from build123d import *

# Parameters (mm, degrees)
BOSS_EXTRUDE1_DEPTH = 80
SHELL1_T            = -3
SKETCH3_W           = 46
SKETCH3_H           = 47
BOSS_EXTRUDE2_DEPTH = 17
SKETCH4_W           = 10.2
SKETCH4_H           = 10.2
CUT_EXTRUDE1_DEPTH  = 20
SKETCH6_W           = 15
SKETCH6_H           = 12.8
CUT_EXTRUDE2_DEPTH  = 3
SKETCH7_W           = 40.4
SKETCH7_H           = 50
CUT_EXTRUDE3_DEPTH  = 5
FILLET1_R           = 4
CUT_EXTRUDE7_DEPTH  = 47
SKETCH13_R          = 1.5
CUT_EXTRUDE8_DEPTH  = 25
SKETCH14_R          = 3.1
CUT_EXTRUDE9_DEPTH  = 2
SKETCH17_W          = 45
SKETCH17_H          = 5
BOSS_EXTRUDE5_DEPTH = 74
CUT_EXTRUDE10_REACH = 126.093
SKETCH18_W          = 54
SKETCH18_H          = 45
CUT_EXTRUDE11_REACH = 126.093
SKETCH19_R          = 1.45
BOSS_EXTRUDE6_DEPTH = 47
SKETCH22_R          = 1.45
CUT_EXTRUDE12_DEPTH = 135.415364765
CUT_EXTRUDE13_REACH = 126.857
SKETCH24_R          = 3.7
SKETCH24_W          = 2
SKETCH24_H          = 3
BOSS_EXTRUDE7_DEPTH = 74
SKETCH27_R          = 1.5
CUT_EXTRUDE14_DEPTH = 10
CUT_EXTRUDE15_START = -3
CUT_EXTRUDE15_DEPTH = 32
CUT_EXTRUDE16_DEPTH = 30
BOSS_EXTRUDE8_DEPTH = 20
SKETCH31_R          = 1.5
CUT_EXTRUDE17_DEPTH = 123.649786567
CUT_EXTRUDE18_DEPTH = 15
CUT_EXTRUDE19_REACH = 126.093
SKETCH33_W          = 10
SKETCH33_H          = 5
SKETCH34_R          = 1.6
CUT_EXTRUDE20_DEPTH = 135.415364765
CUT_EXTRUDE22_DEPTH = 14


with BuildPart() as part:
    # Sketch2 → Boss-Extrude1 (new body)
    with BuildSketch(Plane(origin=(0, 0, 0), x_dir=(0, 0, -1), z_dir=(1, 0, 0))):
        Polygon((-27.320490368, 20.998248687), (-27.320490368, -29.001751313), (12.679509632, -29.001751313), (12.679509632, -48.511383538), (27.679509632, -48.511383538), (82.679509632, 0.998248687), (82.679509632, 20.998248687), align=None)
    extrude(amount=BOSS_EXTRUDE1_DEPTH)

    # Shell1
    shell1_openings = [part.faces().sort_by_distance(p)[0] for p in [
        (40, 20.998248687, -27.679509632),
    ]]
    offset(amount=SHELL1_T, openings=shell1_openings, kind=Kind.INTERSECTION)

    # Sketch3 → Boss-Extrude2 (add)
    with BuildSketch(Plane(origin=(0, 0, 24.320490368), x_dir=(-1, 0, 0), z_dir=(0, 0, -1))):
        with Locations((-40, -2.501751313)):
            Rectangle(SKETCH3_W, SKETCH3_H)
    extrude(amount=BOSS_EXTRUDE2_DEPTH)

    # Sketch4 → Cut-Extrude1 (cut)
    with BuildSketch(Plane.XY.offset(27.320490368)):
        with Locations((40, -4.001751313)):
            Rectangle(SKETCH4_W, SKETCH4_H)
    extrude(amount=-CUT_EXTRUDE1_DEPTH, mode=Mode.SUBTRACT)

    # Sketch6 → Cut-Extrude2 (cut)
    with BuildSketch(Plane.XZ.offset(29.001751313)):
        with Locations((40, 0.920490368)):
            Rectangle(SKETCH6_W, SKETCH6_H)
    extrude(amount=-CUT_EXTRUDE2_DEPTH, mode=Mode.SUBTRACT)

    # Sketch7 → Cut-Extrude3 (cut)
    with BuildSketch(Plane.XY.offset(27.320490368)):
        with Locations((40, -4.001751313)):
            Rectangle(SKETCH7_W, SKETCH7_H)
    extrude(amount=-CUT_EXTRUDE3_DEPTH, mode=Mode.SUBTRACT)

    # Fillet1
    fillet1_edges = [part.edges().sort_by_distance(p)[0] for p in [
        (80, -4.001751313, 27.320490368),
        (19.8, -4.001751313, 27.320490368),
        (0, -4.001751313, 27.320490368),
        (60.2, -4.001751313, 27.320490368),
    ]]
    fillet(fillet1_edges, radius=FILLET1_R)

    # Sketch12 → Cut-Extrude7 (cut)
    with BuildSketch(Plane(origin=(0, 20.998248687, 0), x_dir=(1, 0, 0), z_dir=(0, 1, 0))):
        Polygon((33, -7.320490368), (19.8, -12.320490368), (17, -24.320490368), (17, -7.320490368), align=None)
        Polygon((47, -7.320490368), (63, -7.320490368), (63, -24.320490368), (60.2, -12.320490368), align=None)
    extrude(amount=-CUT_EXTRUDE7_DEPTH, mode=Mode.SUBTRACT)

    # Sketch13 → Cut-Extrude8 (cut)
    with BuildSketch(Plane(origin=(0, 20.998248687, 0), x_dir=(1, 0, 0), z_dir=(0, 1, 0))):
        with Locations(Location((26, -17.320490368, 0), (0, 0, 270))):
            Circle(SKETCH13_R)
        with Locations(Location((54, -17.320490368, 0), (0, 0, 270))):
            Circle(SKETCH13_R)
    extrude(amount=-CUT_EXTRUDE8_DEPTH, mode=Mode.SUBTRACT)

    # Sketch14 → Cut-Extrude9 (cut)
    with BuildSketch(Plane(origin=(0, 20.998248687, 0), x_dir=(1, 0, 0), z_dir=(0, 1, 0))):
        with Locations(Location((26, -17.320490368, 0), (0, 0, 270))):
            Circle(SKETCH14_R)
        with Locations(Location((54, -17.320490368, 0), (0, 0, 270))):
            Circle(SKETCH14_R)
    extrude(amount=-CUT_EXTRUDE9_DEPTH, mode=Mode.SUBTRACT)

    # Sketch17 → Boss-Extrude5 (add)
    with BuildSketch(Plane.ZY.offset(-77)):
        with Locations((-23.179509632, -4.501751313)):
            Rectangle(SKETCH17_W, SKETCH17_H)
    extrude(amount=BOSS_EXTRUDE5_DEPTH)

    # Sketch18 → Cut-Extrude10 (cut, up to next)
    with BuildSketch(Plane(origin=(0, -2.001751313, 0), x_dir=(1, 0, 0), z_dir=(0, 1, 0)), mode=Mode.PRIVATE) as cut_extrude10_sk1:
        with Locations((40, 23.179509632)):
            Rectangle(SKETCH18_W, SKETCH18_H)
    cut_extrude10_tool1 = extrude(cut_extrude10_sk1.sketch, amount=-CUT_EXTRUDE10_REACH, mode=Mode.PRIVATE) & part.part
    add(cut_extrude10_tool1.solids().sort_by_distance((40, -2.001751, -23.17951))[0], mode=Mode.SUBTRACT)

    # Sketch19 → Cut-Extrude11 (cut, up to next)
    with BuildSketch(Plane(origin=(0, -2.001751313, 0), x_dir=(1, 0, 0), z_dir=(0, 1, 0)), mode=Mode.PRIVATE) as cut_extrude11_sk1:
        with Locations(Location((72, 37.179509632, 0), (0, 0, 270))):
            Circle(SKETCH19_R)
    cut_extrude11_tool1 = extrude(cut_extrude11_sk1.sketch, amount=-CUT_EXTRUDE11_REACH, mode=Mode.PRIVATE) & part.part
    # Sketch19 → Cut-Extrude11 (cut, up to next)
    with BuildSketch(Plane(origin=(0, -2.001751313, 0), x_dir=(1, 0, 0), z_dir=(0, 1, 0)), mode=Mode.PRIVATE) as cut_extrude11_sk2:
        with Locations(Location((72, 6.179509632, 0), (0, 0, 270))):
            Circle(SKETCH19_R)
    cut_extrude11_tool2 = extrude(cut_extrude11_sk2.sketch, amount=-CUT_EXTRUDE11_REACH, mode=Mode.PRIVATE) & part.part
    # Sketch19 → Cut-Extrude11 (cut, up to next)
    with BuildSketch(Plane(origin=(0, -2.001751313, 0), x_dir=(1, 0, 0), z_dir=(0, 1, 0)), mode=Mode.PRIVATE) as cut_extrude11_sk3:
        with Locations(Location((8, 33.179509632, 0), (0, 0, 270))):
            Circle(SKETCH19_R)
    cut_extrude11_tool3 = extrude(cut_extrude11_sk3.sketch, amount=-CUT_EXTRUDE11_REACH, mode=Mode.PRIVATE) & part.part
    # Sketch19 → Cut-Extrude11 (cut, up to next)
    with BuildSketch(Plane(origin=(0, -2.001751313, 0), x_dir=(1, 0, 0), z_dir=(0, 1, 0)), mode=Mode.PRIVATE) as cut_extrude11_sk4:
        with Locations(Location((8, 6.179509632, 0), (0, 0, 270))):
            Circle(SKETCH19_R)
    cut_extrude11_tool4 = extrude(cut_extrude11_sk4.sketch, amount=-CUT_EXTRUDE11_REACH, mode=Mode.PRIVATE) & part.part
    add(cut_extrude11_tool1.solids().sort_by_distance((72, -2.001751, -37.17951))[0], mode=Mode.SUBTRACT)
    add(cut_extrude11_tool2.solids().sort_by_distance((72, -2.001751, -6.17951))[0], mode=Mode.SUBTRACT)
    add(cut_extrude11_tool3.solids().sort_by_distance((8, -2.001751, -33.17951))[0], mode=Mode.SUBTRACT)
    add(cut_extrude11_tool4.solids().sort_by_distance((8, -2.001751, -6.17951))[0], mode=Mode.SUBTRACT)

    # Sketch21 → Boss-Extrude6 (add)
    with BuildSketch(Plane(origin=(0, -26.001751313, 0), x_dir=(1, 0, 0), z_dir=(0, 1, 0))):
        Polygon((3, -24.320490368), (3, -14.320490368), (19.333333333, -14.320490368), (17, -24.320490368), align=None)
    extrude(amount=BOSS_EXTRUDE6_DEPTH)

    # Sketch22 → Cut-Extrude12 (cut, through all)
    with BuildSketch(Plane(origin=(0, 20.998248687, 0), x_dir=(1, 0, 0), z_dir=(0, 1, 0))):
        with Locations(Location((10, -19.320490368, 0), (0, 0, 270))):
            Circle(SKETCH22_R)
    extrude(amount=-CUT_EXTRUDE12_DEPTH, mode=Mode.SUBTRACT)

    # Sketch24 → Cut-Extrude13 (cut, up to next)
    with BuildSketch(Plane(origin=(80, 0, 0), x_dir=(0, 0, -1), z_dir=(1, 0, 0)), mode=Mode.PRIVATE) as cut_extrude13_sk1:
        with Locations((26.679509632, -30.511383538)):
            Circle(SKETCH24_R)
    cut_extrude13_tool1 = extrude(cut_extrude13_sk1.sketch, amount=-CUT_EXTRUDE13_REACH, mode=Mode.PRIVATE) & part.part
    # Sketch24 → Cut-Extrude13 (cut, up to next)
    with BuildSketch(Plane(origin=(80, 0, 0), x_dir=(0, 0, -1), z_dir=(1, 0, 0)), mode=Mode.PRIVATE) as cut_extrude13_sk2:
        with Locations((34.379509632, -30.511383538)):
            Rectangle(SKETCH24_W, SKETCH24_H)
    cut_extrude13_tool2 = extrude(cut_extrude13_sk2.sketch, amount=-CUT_EXTRUDE13_REACH, mode=Mode.PRIVATE) & part.part
    add(cut_extrude13_tool1.solids().sort_by_distance((80, -30.511384, -26.67951))[0], mode=Mode.SUBTRACT)
    add(cut_extrude13_tool2.solids().sort_by_distance((80, -30.511384, -34.37951))[0], mode=Mode.SUBTRACT)

    # Sketch26 → Boss-Extrude7 (add)
    with BuildSketch(Plane(origin=(3, 0, 0), x_dir=(0, 0, -1), z_dir=(1, 0, 0))):
        Polygon((79.679509632, 2.334161996), (63.679509632, 2.334161996), (63.679509632, -12.068640106), align=None)
    extrude(amount=BOSS_EXTRUDE7_DEPTH)

    # Sketch27 → Cut-Extrude14 (cut)
    with BuildSketch(Plane(origin=(0, 2.334161996, 0), x_dir=(1, 0, 0), z_dir=(0, 1, 0))):
        with Locations(Location((6, 76.679509632, 0), (0, 0, 270))):
            Circle(SKETCH27_R)
        with Locations(Location((74, 76.679509632, 0), (0, 0, 270))):
            Circle(SKETCH27_R)
    extrude(amount=-CUT_EXTRUDE14_DEPTH, mode=Mode.SUBTRACT)

    # Sketch28 → Cut-Extrude15 (cut)
    with BuildSketch(Plane(origin=(0, 2.334161996, 0), x_dir=(1, 0, 0), z_dir=(0, 1, 0)).offset(CUT_EXTRUDE15_START)):
        Polygon((74, 79.929509632), (71.185417438, 78.304509632), (71.185417438, 75.054509632), (74, 73.429509632), (76.814582562, 75.054509632), (76.814582562, 78.304509632), align=None)
        Polygon((6, 73.429509632), (8.814582562, 75.054509632), (8.814582562, 78.304509632), (6, 79.929509632), (3.185417438, 78.304509632), (3.185417438, 75.054509632), align=None)
    extrude(amount=-CUT_EXTRUDE15_DEPTH, mode=Mode.SUBTRACT)

    # Sketch29 → Cut-Extrude16 (cut)
    with BuildSketch(Plane.XZ.offset(29.001751313)):
        Polygon((7.185417438, 17.695490368), (10, 16.070490368), (12.814582562, 17.695490368), (12.814582562, 20.945490368), (10, 22.570490368), (7.185417438, 20.945490368), align=None)
    extrude(amount=-CUT_EXTRUDE16_DEPTH, mode=Mode.SUBTRACT)

    # Sketch30 → Boss-Extrude8 (add)
    with BuildSketch(Plane(origin=(0, -26.001751313, 0), x_dir=(1, 0, 0), z_dir=(0, 1, 0))):
        Polygon((77, -24.320490368), (63, -24.320490368), (60.2, -12.320490368), (77, -12.320490368), align=None)
    extrude(amount=BOSS_EXTRUDE8_DEPTH)

    # Sketch31 → Cut-Extrude17 (cut, through all)
    with BuildSketch(Plane(origin=(0, -6.001751313, 0), x_dir=(1, 0, 0), z_dir=(0, 1, 0))):
        with Locations(Location((72, -21.320490368, 0), (0, 0, 270))):
            Circle(SKETCH31_R)
    extrude(amount=-CUT_EXTRUDE17_DEPTH, mode=Mode.SUBTRACT)

    # Sketch32 → Cut-Extrude18 (cut)
    with BuildSketch(Plane.XZ.offset(29.001751313)):
        Polygon((72, 24.570490368), (69.185417438, 22.945490368), (69.185417438, 19.695490368), (72, 18.070490368), (74.814582562, 19.695490368), (74.814582562, 22.945490368), align=None)
    extrude(amount=-CUT_EXTRUDE18_DEPTH, mode=Mode.SUBTRACT)

    # Sketch33 → Cut-Extrude19 (cut, up to next)
    with BuildSketch(Plane(origin=(0, -2.001751313, 0), x_dir=(1, 0, 0), z_dir=(0, 1, 0)), mode=Mode.PRIVATE) as cut_extrude19_sk1:
        with Locations((72, 43.179509632)):
            Rectangle(SKETCH33_W, SKETCH33_H)
    cut_extrude19_tool1 = extrude(cut_extrude19_sk1.sketch, amount=-CUT_EXTRUDE19_REACH, mode=Mode.PRIVATE) & part.part
    add(cut_extrude19_tool1.solids().sort_by_distance((72, -2.001751, -43.17951))[0], mode=Mode.SUBTRACT)

    # Sketch34 → Cut-Extrude20 (cut, through all)
    with BuildSketch(Plane(origin=(0, 20.998248687, 0), x_dir=(1, 0, 0), z_dir=(0, 1, 0))):
        with Locations(Location((40, -17.320490368, 0), (0, 0, 270))):
            Circle(SKETCH34_R)
    extrude(amount=-CUT_EXTRUDE20_DEPTH, mode=Mode.SUBTRACT)

    # Sketch36 → Cut-Extrude22 (cut)
    with BuildSketch(Plane.XZ.offset(29.001751313)):
        Polygon((38.375, 20.13507293), (36.75, 17.320490368), (38.375, 14.505907805), (41.625, 14.505907805), (43.25, 17.320490368), (41.625, 20.13507293), align=None)
    extrude(amount=-CUT_EXTRUDE22_DEPTH, mode=Mode.SUBTRACT)


solid = part.part
Source: CAD feature listing. Evaluate the final solid. Frame: model axes, mm. A direction names the side the tool comes from. Round coordinates to 2 decimals unless told otherwise and drop trailing zeros. Write each loop counter-clockwise with the first axis right and the second up, starting at its lowest first coordinate (ties: lowest second). Pieces come first, ordered by that corner, then holes. Notation, with made-up numbers: M -27.75,-13.75 L -19.75,-13.75 A17 cw -19.75,2.25 Z; hole C 4,59 d1. An arc over 180 degrees is marked long. One line per item, written item: value. Start each with the question number.
Item 1: Mould query, pull axis Y, two halves, no side actions, for faces 1 (the flat face through (13, -4, -23)), 2 (the flat face through (8, -2.002, -23)), 3 (the flat face through (79, -31, -33.38)). Classes: pulls with the +Y half, pulls with the -Y half, needs draft (parallel to the pull), parting line crosses it, or undercut.
Item 2: Ray query, L1, parallel to Z at x = 74, y = 1.5; L2, parallel to X at y = 8, z = -72.5; L3, parallel to Z at x = 16, y = 7. Return the intervals inside material, ascending. Write a range as from..to.
Item 3: Pin query (flat end, axial travel): pin 1 (4.5 mm diameter, centred on x = 72, z = -6.18, fed in from +Y); pin 2 (1 mm diameter, centred on x = 39, y = -25, fed in from +Z); pin 3 (2.5 mm diameter, centred on x = 72, z = 21.32, fed in from -Y); pin 4 (4 mm diameter, centred on x = 40, z = 17.32, fed in from +Y). Return the tip coordinate at first contact, or that it passes through.
Item 4: Section query A-A (x = 40). State how many separate pieces and enclosed holes the cut face has, plus the area to 3 significant figures.
Item 5: Section query C-C (y = 15). Return the cut outline in (x, z).
Item 6: Section query D-D (z = -20.5). Return the cut outline in (x, y).
Item 7: Set-up query: faces 4 (the flat face through (4.573, -3.95, -74.253)), 5 (the flat face through (8, -7.002, -23)), 6 (the flat face through (39, -5, -63.68)), 7 (the cylindrical face through (78.521, -30.349, -22.983)). Return all of +Z, -Z, +X, -X, +Y, -Y with unobstructed straight access to the full face (end or side cutting, diameter ignored); none if empty.
Item 8: Section query B-B (z = 1). Return the cut outline in (x, y).
Result set:
1. face 1: needs draft
1. face 2: pulls with the +Y half
1. face 3: undercut
2. L1: z = -82.68..-78.18, -75.18..-63.68, 24.32..27.32
2. L2: x = 0..3, 77..80
2. L3: z = -82.68..-79.68, 14.32..27.32
3. pin 1: stops at y = -2
3. pin 2: stops at z = 22.32
3. pin 3: passes through
3. pin 4: stops at y = 21
4. separate pieces: 5
4. enclosed holes: 0
4. area: 951 mm²
5. outline: M 0,-82.68 L 80,-82.68 L 80,23.32 A4 ccw 76,27.32 L 64.2,27.32 A4 ccw 60.2,23.32 L 60.2,22.32 L 19.8,22.32 L 19.8,23.32 A4 ccw 15.8,27.32 L 4,27.32 A4 ccw 0,23.32 Z; hole M 3,-79.68 L 77,-79.68 L 77,24.32 L 63,24.32 L 60.2,12.32 L 47,7.32 L 33,7.32 L 19.8,12.32 L 19.33,14.32 L 3,14.32 Z; hole C 10,19.32 d2.9; hole C 26,17.32 d3; hole C 40,17.32 d3.2; hole C 54,17.32 d3
6. outline: M 0,-48.51 L 80,-48.51 L 80,21 L 77,21 L 77,-2 L 67,-2 L 67,-7 L 77,-7 L 77,-45.51 L 3,-45.51 L 3,-7 L 13,-7 L 13,-2 L 3,-2 L 3,21 L 0,21 Z
7. face 4: -Y
7. face 5: none
7. face 6: +Y
7. face 7: +X
8. outline: M 0,-29 L 32.5,-29 L 32.5,-26 L 3,-26 L 3,21 L 0,21 Z; M 47.5,-29 L 80,-29 L 80,21 L 77,21 L 77,-26 L 47.5,-26 Z
